Verification items for this drawing (mm, ordinates from the low corner). A direction names the side the tool comes from. Give positions to 0.01 mm unless a question says otherwise; leave off trailing zeros. Write each loop counter-clockwise with the first axis right and the second up, starting at its lowest first coordinate (ties: lowest second). Pieces come first, ordered by that corner, then holes. Notation, with made-up numbers: (44, 88) -> (68, 88) arc R16 cw to (68, 119) -> close; hole circle Ø11 at (53, 70). An arc over 180 degrees is marked (long way). One line per item, written item: value.
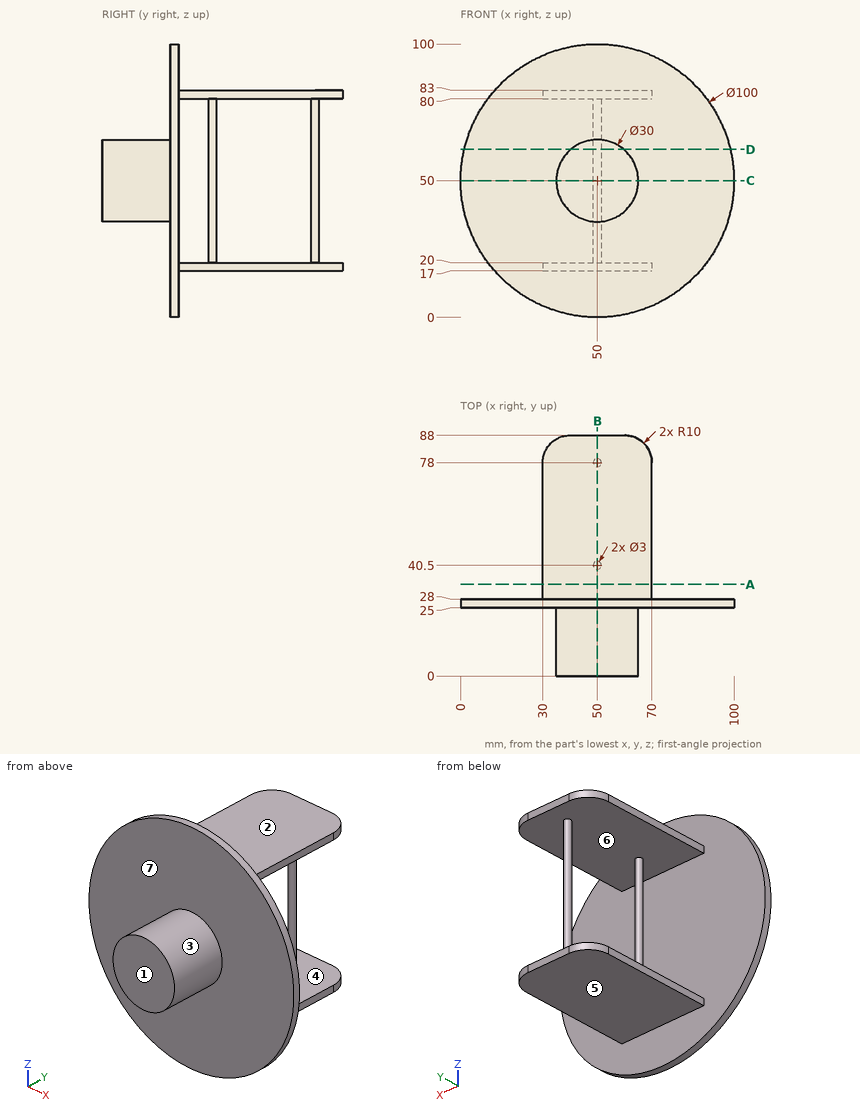
1) Sectioned sample at B-B on x = 50. Record the cut outline in (y, z), plus the area to 3 significant figures.
Verdict:
outline: (0, 35) -> (25, 35) -> (25, 0) -> (28, 0) -> (28, 17) -> (88, 17) -> (88, 20) -> (79.5, 20) -> (79.5, 80) -> (88, 80) -> (88, 83) -> (28, 83) -> (28, 100) -> (25, 100) -> (25, 65) -> (0, 65) -> close; hole (28, 20) -> (39, 20) -> (39, 80) -> (28, 80) -> close; hole (42, 20) -> (76.5, 20) -> (76.5, 80) -> (42, 80) -> close
area: 1,770 mm^2
2) Depth check by flat-ended pin: pin 1 Ø2 at (y, z) = (23.5, 88) entering from +X; pin 2 Ø0.9 at (y, z) = (54, 81) entering from +X; pin 3 Ø2.5 at (y, z) = (45.5, 18) entering from -X; pin 4 Ø12 at (x, z) = (70.5, 52) entering from +Y. Enter the tip coordinate at first touch or a pass-through.
Verdict:
pin 1: through
pin 2: x = 70
pin 3: x = 30
pin 4: y = 28
3) Scan lines: probe 1 along Z at (x, y) = (59, 64); probe 2 along X at (y, z) = (78, 60.5); probe 3 along Y at (x, z) = (52, 39). Record each from-to range of solid material in increasing order.
Verdict:
probe 1: 17 to 20, 80 to 83
probe 2: 48.5 to 51.5
probe 3: 0 to 28
4) Sectioned sample at C-C on z = 50. Record the cut outline in (x, y), plus the area to 3 significant figures.
Verdict:
outline: (0, 25) -> (35, 25) -> (35, 0) -> (65, 0) -> (65, 25) -> (100, 25) -> (100, 28) -> (0, 28) -> close; circle Ø3 at (50, 40.5); circle Ø3 at (50, 78)
area: 1,060 mm^2
5) Sectioned sample at A-A on y = 33.5. Record the cut outline in (x, z), plus the area to 3 significant figures.
Verdict:
outline: (30, 17) -> (70, 17) -> (70, 20) -> (30, 20) -> close; (30, 80) -> (70, 80) -> (70, 83) -> (30, 83) -> close
area: 240 mm^2
6) Mould release check, pull along Z, two halves, no side actions. Record for the marked faces 4, 5, 6 and 7: released by +Z, released by -Z, zero draft, split by the parting line, or undercut.
Verdict:
face 4: undercut
face 5: released by -Z
face 6: undercut
face 7: zero draft
7) Sectioned sample at D-D on z = 61.5. Record the cut outline in (x, y).
Verdict:
outline: (1.34, 25) -> (40.37, 25) -> (40.37, 0) -> (59.63, 0) -> (59.63, 25) -> (98.66, 25) -> (98.66, 28) -> (1.34, 28) -> close; circle Ø3 at (50, 40.5); circle Ø3 at (50, 78)
8) Tool access check on the marked faces 1, 2 and 3. Record the directions out of +Z, -Z, +X, -X, +Y, -Y that give a thin tool (end or side, any length) a straight path to the whole face; none if there is none.
Verdict:
face 1: +Z, -Z, +X, -X, -Y
face 2: +Z, +X, -X, +Y
face 3: -Y
